Check sheet for the modelled part. Datum: model origin and axes. Units: mm. Give positions to 0.01 mm unless a question says otherwise; leave off trailing zeros.
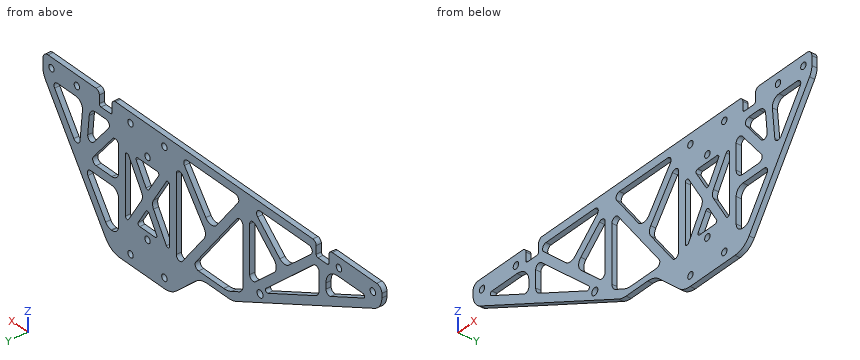
from build123d import *

# Parameters (mm, degrees)
SKETCH1_R               = 2.032
BOSS_EXTRUDE1_DEPTH     = 3.175
SKETCH1_3_R             = 2.032
CUT_EXTRUDE2_DEPTH      = 270.126904313
FILLET1_R               = 3.81
FILLET2_R               = 10.16
FILLET3_R               = 12.7
FILLET4_R               = 1.27
FILLET5_R               = 2.54
FILLET6_R               = 5.08
FILLET7_R               = 12.7
FILLET10_R              = 8.89
CUT_EXTRUDE5_DEPTH      = 270.126904313
CUT_EXTRUDE5_DEPTH_BACK = 270.126904313
FILLET11_R              = 12.7
SKETCH2_W               = 9.525
SKETCH2_H               = 8.89
CUT_EXTRUDE3_DEPTH      = 270.126904313
FILLET8_R               = 1.27
FILLET9_R               = 2.54
SKETCH3_R               = 2.286
CUT_EXTRUDE4_DEPTH      = 3.175


with BuildPart() as part:
    # Sketch1 → Boss-Extrude1 (new body)
    with BuildSketch(Plane(origin=(0, 0, 0), x_dir=(1, 0, 0), z_dir=(0, 1, 0))):
        Polygon((0, 0), (254, 0), (254, 12.7), (203.2, 88.9), (152.4, 88.9), (0, 12.7), align=None)
        with Locations(Location((6.773333333, 6.35, 0), (0, 0, 270))):
            Circle(SKETCH1_R, mode=Mode.SUBTRACT)
        with Locations(Location((32.173333333, 6.35, 0), (0, 0, 270))):
            Circle(SKETCH1_R, mode=Mode.SUBTRACT)
        with Locations(Location((228.6, 6.35, 0), (0, 0, 270))):
            Circle(SKETCH1_R, mode=Mode.SUBTRACT)
        with Locations(Location((247.65, 6.35, 0), (0, 0, 270))):
            Circle(SKETCH1_R, mode=Mode.SUBTRACT)
        with Locations(Location((162.983333333, 82.55, 0), (0, 0, 270))):
            Circle(SKETCH1_R, mode=Mode.SUBTRACT)
        with Locations(Location((188.383333333, 82.55, 0), (0, 0, 270))):
            Circle(SKETCH1_R, mode=Mode.SUBTRACT)
    extrude(amount=BOSS_EXTRUDE1_DEPTH)

    # Sketch1<3> → Cut-Extrude2 (cut, through all)
    with BuildSketch(Plane(origin=(0, 0, 0), x_dir=(1, 0, 0), z_dir=(0, 1, 0))):
        Polygon((8.819225326, 11.43), (41.91, 11.43), (41.91, 27.975387337), align=None)
        Polygon((73.025, 27.993892654), (48.195281614, 5.08), (97.854718386, 5.08), align=None)
        Polygon((46.99, 30.515387337), (46.99, 10.88031823), (93.426011301, 53.733392988), align=None)
        with Locations(Location((188.383333333, 6.35, 0), (0, 0, 270))):
            Circle(SKETCH1_3_R)
        Polygon((104.756949825, 5.08), (150.936383508, 5.08), (127.846666667, 36.362842172), align=None)
        with Locations(Location((162.983333333, 6.35, 0), (0, 0, 270))):
            Circle(SKETCH1_3_R)
        Polygon((99.06, 52.020069107), (76.770281614, 31.450193669), (99.06, 10.88031823), align=None)
        Polygon((142.499954937, 64.77), (115.499225326, 64.77), (104.14, 59.090387337), (104.14, 12.79844815), align=None)
        Polygon((223.00729992, 50.03094988), (205.561266507, 76.2), (197.273333333, 76.2), (197.273333333, 50.03094988), align=None)
        Polygon((131.003616492, 40.64), (154.093333333, 9.357157828), (154.093333333, 71.922842172), align=None)
        Polygon((197.273333333, 44.95094988), (197.273333333, 16.802739743), (219.463857142, 44.95094988), align=None)
        Polygon((166.148656896, 23.622), (185.218009771, 23.622), (175.683333333, 39.513127396), align=None)
        Polygon((178.645456896, 44.45), (192.193333333, 21.870205938), (192.193333333, 67.029794062), align=None)
        Polygon((221.333484531, 39.117053196), (201.508910253, 13.97), (218.885586813, 13.97), align=None)
        Polygon((223.865972381, 12.7), (247.89459984, 12.7), (226.927485283, 44.150671836), align=None)
        Polygon((159.173333333, 67.029794062), (159.173333333, 21.870205938), (172.721209771, 44.45), align=None)
        Polygon((175.683333333, 49.386872604), (183.694009771, 62.738), (167.672656896, 62.738), align=None)
        with Locations(Location((175.683333333, 19.05, 0), (0, 0, 270))):
            Circle(SKETCH1_3_R)
        with Locations(Location((175.683333333, 67.31, 0), (0, 0, 270))):
            Circle(SKETCH1_3_R)
    extrude(amount=CUT_EXTRUDE2_DEPTH, mode=Mode.SUBTRACT)

    # Fillet1
    fillet1_edges = [part.edges().sort_by_distance(p)[0] for p in [
        (0, 1.5875, 0),
        (254, 1.5875, 0),
    ]]
    fillet(fillet1_edges, radius=FILLET1_R)

    # Fillet2
    fillet2_edges = [part.edges().sort_by_distance(p)[0] for p in [
        (254, 1.5875, -12.7),
        (0, 1.5875, -12.7),
    ]]
    fillet(fillet2_edges, radius=FILLET2_R)

    # Fillet3
    fillet3_edges = [part.edges().sort_by_distance(p)[0] for p in [
        (203.2, 1.5875, -88.9),
        (152.4, 1.5875, -88.9),
    ]]
    fillet(fillet3_edges, radius=FILLET3_R)

    # Fillet4
    fillet4_edges = [part.edges().sort_by_distance(p)[0] for p in [
        (175.683333333, 1.5875, -39.513127396),
        (166.148656896, 1.5875, -23.622),
        (185.218009771, 1.5875, -23.622),
        (159.173333333, 1.5875, -67.029794062),
        (159.173333333, 1.5875, -21.870205938),
        (183.694009771, 1.5875, -62.738),
        (167.672656896, 1.5875, -62.738),
        (175.683333333, 1.5875, -49.386872604),
        (8.819225326, 1.5875, -11.43),
        (192.193333333, 1.5875, -67.029794062),
        (192.193333333, 1.5875, -21.870205938),
        (93.426011301, 1.5875, -53.733392988),
    ]]
    fillet(fillet4_edges, radius=FILLET4_R)

    # Fillet5
    fillet5_edges = [part.edges().sort_by_distance(p)[0] for p in [
        (247.89459984, 1.5875, -12.7),
        (226.927485283, 1.5875, -44.150671836),
        (221.333484531, 1.5875, -39.117053196),
        (201.508910253, 1.5875, -13.97),
        (41.91, 1.5875, -27.975387337),
        (99.06, 1.5875, -52.020069107),
        (99.06, 1.5875, -10.88031823),
        (97.854718386, 1.5875, -5.08),
        (48.195281614, 1.5875, -5.08),
        (150.936383508, 1.5875, -5.08),
        (104.756949825, 1.5875, -5.08),
        (142.499954937, 1.5875, -64.77),
        (104.14, 1.5875, -12.79844815),
        (223.00729992, 1.5875, -50.03094988),
        (197.273333333, 1.5875, -16.802739743),
        (219.463857142, 1.5875, -44.95094988),
        (154.093333333, 1.5875, -9.357157828),
        (154.093333333, 1.5875, -71.922842172),
        (46.99, 1.5875, -10.88031823),
    ]]
    fillet(fillet5_edges, radius=FILLET5_R)

    # Fillet6
    fillet6_edges = [part.edges().sort_by_distance(p)[0] for p in [
        (223.865972381, 1.5875, -12.7),
        (172.721209771, 1.5875, -44.45),
        (218.885586813, 1.5875, -13.97),
        (76.770281614, 1.5875, -31.450193669),
        (73.025, 1.5875, -27.993892654),
        (127.846666667, 1.5875, -36.362842172),
        (104.14, 1.5875, -59.090387337),
        (178.645456896, 1.5875, -44.45),
        (197.273333333, 1.5875, -50.03094988),
        (205.561266507, 1.5875, -76.2),
        (197.273333333, 1.5875, -76.2),
        (197.273333333, 1.5875, -44.95094988),
        (131.003616492, 1.5875, -40.64),
        (46.99, 1.5875, -30.515387337),
    ]]
    fillet(fillet6_edges, radius=FILLET6_R)

    # Fillet7
    fillet7_edges = [part.edges().sort_by_distance(p)[0] for p in [
        (115.499225326, 1.5875, -64.77),
    ]]
    fillet(fillet7_edges, radius=FILLET7_R)

    # Fillet10
    fillet10_edges = [part.edges().sort_by_distance(p)[0] for p in [
        (41.91, 1.5875, -11.43),
    ]]
    fillet(fillet10_edges, radius=FILLET10_R)

    # Sketch4 → Cut-Extrude5 (cut, two sides: drawn at the far end of the back side and taken through both)
    with BuildSketch(Plane(origin=(0, 3.175, 0), x_dir=(1, 0, 0), z_dir=(0, 1, 0)).offset(-CUT_EXTRUDE5_DEPTH_BACK)):
        with BuildLine():
            Line((111.76, 68.58), (118.49728864, 68.58))
            Line((118.49728864, 68.58), (135.969082876, 68.58))
            Line((135.969082876, 68.58), (157.79217598, 88.9))
            Line((157.79217598, 88.9), (155.398063314, 88.9))
            ThreePointArc((155.398063314, 88.9), (152.480201223, 88.560262166), (149.718450651, 87.559225326))
            Line((149.718450651, 87.559225326), (111.76, 68.58))
        make_face()
    extrude(amount=CUT_EXTRUDE5_DEPTH + CUT_EXTRUDE5_DEPTH_BACK, mode=Mode.SUBTRACT)

    # Fillet11
    fillet11_edges = [part.edges().sort_by_distance(p)[0] for p in [
        (157.79217598, 1.5875, -88.9),
        (135.969082876, 1.5875, -68.58),
        (111.76, 1.5875, -68.58),
    ]]
    fillet(fillet11_edges, radius=FILLET11_R)

    # Sketch2 → Cut-Extrude3 (cut, through all)
    with BuildSketch(Plane(origin=(0, 3.175, 0), x_dir=(1, 0, 0), z_dir=(0, 1, 0))):
        with Locations((44.45, 4.445)):
            Rectangle(SKETCH2_W, SKETCH2_H)
        with Locations((207.01, 4.445)):
            Rectangle(SKETCH2_W, SKETCH2_H)
    extrude(amount=-CUT_EXTRUDE3_DEPTH, mode=Mode.SUBTRACT)

    # Fillet8
    fillet8_edges = [part.edges().sort_by_distance(p)[0] for p in [
        (39.6875, 1.5875, -8.89),
        (49.2125, 1.5875, -8.89),
        (202.2475, 1.5875, -8.89),
        (211.7725, 1.5875, -8.89),
    ]]
    fillet(fillet8_edges, radius=FILLET8_R)

    # Fillet9
    fillet9_edges = [part.edges().sort_by_distance(p)[0] for p in [
        (39.6875, 1.5875, 0),
        (49.2125, 1.5875, 0),
        (202.2475, 1.5875, 0),
        (211.7725, 1.5875, 0),
    ]]
    fillet(fillet9_edges, radius=FILLET9_R)

    # Sketch3 → Cut-Extrude4 (cut)
    with BuildSketch(Plane(origin=(0, 3.175, 0), x_dir=(1, 0, 0), z_dir=(0, 1, 0))):
        with Locations(Location((91.288247909, 53.284636108, 0), (0, 0, 270))):
            Circle(SKETCH3_R)
    extrude(amount=-CUT_EXTRUDE4_DEPTH, mode=Mode.SUBTRACT)


solid = part.part
1) Depth check by flat-ended pin: pin 1 Ø1 at (x, y) = (43, 1.5) entering from +Z; pin 2 Ø1.6 at (x, y) = (209.5, 1) entering from -Z; pin 3 Ø1 at (y, z) = (1.5, -41.5) entering from +X; pin 4 Ø3.5 at (x, z) = (188.38, -6.35) entering from +Y. Enter the tip coordinate at first touch or a pass-through.
Recorded:
pin 1: stops at z = -8.89
pin 2: stops at z = -80.65
pin 3: stops at x = 235.13
pin 4: passes through
2) Section check A-A, the plane y = 2.4. State how many separate pieces and enclosed holes the cut face has, then the cut area to 3 significant figures.
Recorded:
separate pieces: 1
enclosed holes: 26
area: 8,070 mm2
3) Material ranges on L1, parallel to Z at x = 138, y = 0.3; L2, parallel to Z at x = 175, y = 2.75; L3, parallel to Z at x = 228.6, y = 1.3, recorded low to high.
Recorded:
L1: z = -70.7 to -64.71, -58.67 to -50.12, -31.16 to -22.61, -5.08 to 0
L2: z = -88.9 to -69.22, -65.4 to -62.74, -50.78 to -38.12, -23.62 to -20.96, -17.14 to 0
L3: z = -50.8 to -39.35, -12.77 to -8.38, -4.32 to 0
